from build123d import *

# Parameters (mm, degrees)
CROQUIS1_R              = 20
CROQUIS1_R_2            = 6.5
SALIENTE_EXTRUIR1_DEPTH = 2.5
CROQUIS2_R              = 11.5
CROQUIS2_R_2            = 6.5
SALIENTE_EXTRUIR2_DEPTH = 10
CROQUIS3_R              = 2
CORTAR_EXTRUIR1_DEPTH   = 15


with BuildPart() as part:
    # Croquis1 → Saliente-Extruir1 (new, symmetric)
    with BuildSketch(Plane.XY):
        Circle(CROQUIS1_R)
        Circle(CROQUIS1_R_2, mode=Mode.SUBTRACT)
    extrude(amount=SALIENTE_EXTRUIR1_DEPTH, both=True)

    # Croquis2 → Saliente-Extruir2 (add)
    with BuildSketch(Plane.XY.offset(2.5)):
        Circle(CROQUIS2_R)
        Circle(CROQUIS2_R_2, mode=Mode.SUBTRACT)
    extrude(amount=SALIENTE_EXTRUIR2_DEPTH)

    # Croquis3 → Cortar-Extruir1 (cut, symmetric)
    with BuildSketch(Plane(origin=(0, 0, 0), x_dir=(1, 0, 0), z_dir=(0, 1, 0))):
        with Locations(Location((0, -8, 0), (0, 0, 270))):
            Circle(CROQUIS3_R)
    extrude(amount=CORTAR_EXTRUIR1_DEPTH, both=True, mode=Mode.SUBTRACT)


solid = part.part
Design review of the part built by this model. Coordinates are the model's own, in mm. A direction names the side the tool comes from. Round coordinates to 2 decimals unless told otherwise and drop trailing zeros. Order: outer loops, then holes, each group sorted by start corner. A loop starts at its lowest first (then second) coordinate and runs counter-clockwise, first axis right, second up. Notation, with made-up numbers: M 59,17 L 95,17 A25 ccw 95,36 Z; hole C 74.25,21 d9. An arc over 180 degrees is marked long. Answer as CSV lines item,"result". Start each with the question number.
1) Tool access review of faces 1 (the face through (5, -5, 12.5)), 2 (the face through (-2.493, -11.227, 7.43)): name each direction out of +Z, -Z, +X, -X, +Y, -Y from which nothing blocks a thin tool from reaching the whole face with its end or side.
2) Wall thickness on line 1 along Z through (x, y) = (0, -9); line 2 along Z through (x, y) = (-4.5, 18); line 3 along Y through (x, z) = (5.5, 9): over which ranges is each line inside the solid? List them lowest first. Write a range as [from, to].
3) Add section B-B (x = 0). Give the boundary of the cut face in (y, z), then the cut area to 3 significant figures.
4) For pin 1 Ø1.5 at (x, z) = (-1.5, 5.5) entering from -Y; pin 2 Ø5 at (x, z) = (-5, 9) entering from +Y (3 decimals); pin 3 Ø3 at (y, z) = (-10.5, 9) entering from +X, all flat-tipped, find the tip position at first contact; note any pin that passes through.
5) Add section A-A (y = 0). Give the boundary of the cut face in (x, z).
6) The part is to be moulded in two halves that separate along X. For faces 3 (the face through (-4.336, -19.524, 0.035)), 4 (the face through (-5, 5, -2.5)), 5 (the face through (0, 9, 6)), say which applies: +X half, -X half, draft (parallel to the pull), parting line (faces both ways), or undercut.
7) Add section C-C (z = 8). Give the boundary of the cut face in (x, y).
8) Add section D-D (z = 11.25). Give the boundary of the cut face in (x, y), then the cut area to 3 significant figures.
Resolved:
1,face 1,"+Z, +X, -X, +Y, -Y"
1,face 2,"+Z"
2,line 1,"[-2.5, 6], [10, 12.5]"
2,line 2,"[-2.5, 2.5]"
2,line 3,"[-10.1, -3.46], [3.46, 10.1]"
3,outline,"M -20,-2.5 L -6.5,-2.5 L -6.5,6 L -11.5,6 L -11.5,2.5 L -20,2.5 Z; M -11.5,10 L -6.5,10 L -6.5,12.5 L -11.5,12.5 Z; M 6.5,-2.5 L 20,-2.5 L 20,2.5 L 11.5,2.5 L 11.5,6 L 6.5,6 Z; M 6.5,10 L 11.5,10 L 11.5,12.5 L 6.5,12.5 Z"
3,area,"195 mm^2"
4,pin 1,"y = -11.48"
4,pin 2,"y = 11.225"
4,pin 3,"x = 7.16"
5,outline,"M -20,-2.5 L -6.5,-2.5 L -6.5,12.5 L -11.5,12.5 L -11.5,2.5 L -20,2.5 Z; M 6.5,-2.5 L 20,-2.5 L 20,2.5 L 11.5,2.5 L 11.5,12.5 L 6.5,12.5 Z"
6,face 3,"parting line"
6,face 4,"draft"
6,face 5,"undercut"
7,outline,"M -2,-11.32 L -2,-6.18 A6.5 cw -2,6.18 L -2,11.32 A11.5 ccw Z; M 2,-11.32 A11.5 ccw 2,11.32 L 2,6.18 A6.5 cw 2,-6.18 Z"
8,outline,"C 0,0 d23; hole C 0,0 d13"
8,area,"283 mm^2"
